Can you work these out from the drawing? Everything is in mm from the part's minimum corner. A direction names the side the tool comes from. Round coordinates to 2 decimals unless told otherwise and drop trailing zeros. Write each loop counter-clockwise with the first axis right and the second up, starting at its lowest first coordinate (ties: lowest second). Pieces come first, ordered by that corner, then holes. Notation, with made-up numbers: (-36.5, 34.25) -> (-5.5, 34.25) arc R12 cw to (-5.5, 49.25) -> close; hole circle Ø4 at (37, 25). An arc over 180 degrees is marked (long way). Answer as CSV lines item,"result".
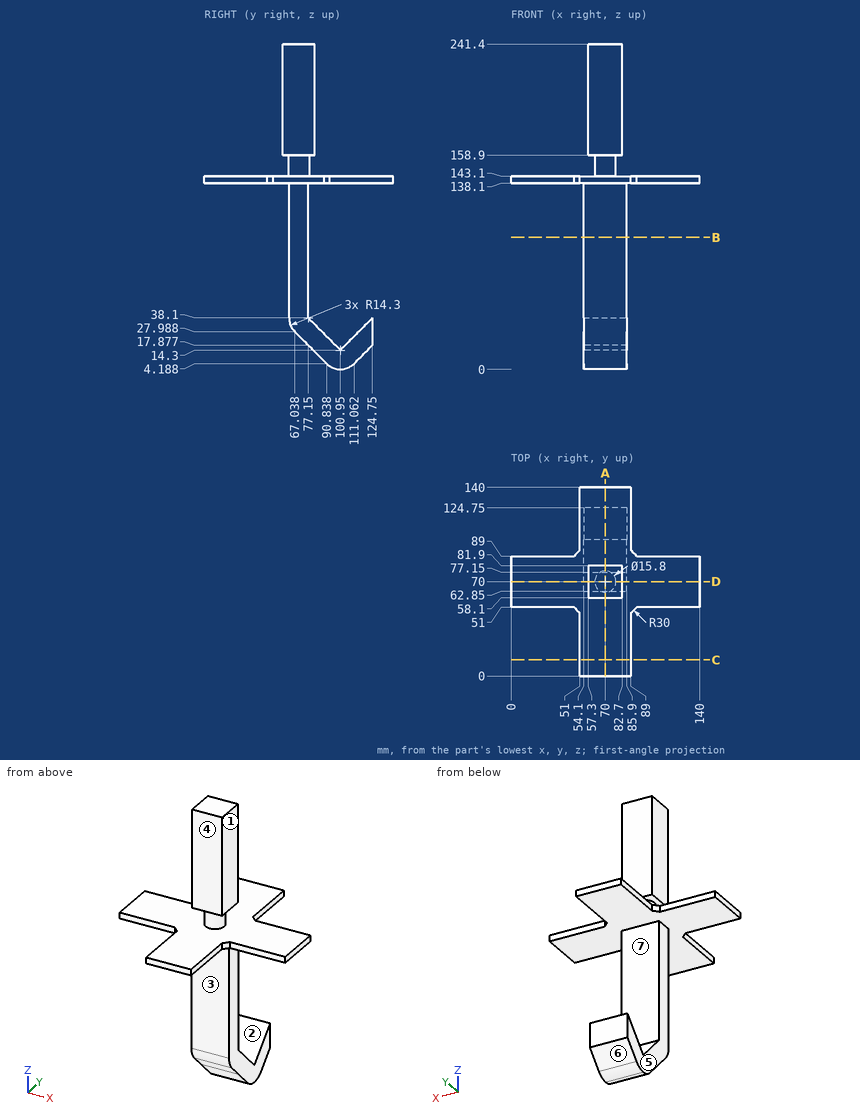
Item 1: If we mould it in two halves opening along Z, with no side actions, what happens to the marked faces 5, 6 and 7? For each: pulls with the +Z half, pulls with the -Z half, needs draft (parallel to the pull), parting line crosses it, or undercut.
Results found:
face 5,"needs draft"
face 6,"pulls with the -Z half"
face 7,"undercut"
Item 2: Will these pins go through, and if not, where does the flat tip stop? pin 1 (6 mm diameter, centred on y = 62, z = 43.5, fed in from +X); pin 2 (4 mm diameter, centred on x = 50.5, y = 20.5, fed in from -Z); pin 3 (4 mm diameter, centred on y = 127, z = 140.5, fed in from -X).
Results found:
pin 1,"stops at x = 85.9"
pin 2,"stops at z = 138.1"
pin 3,"stops at x = 51"
Item 3: Suppose I cut it at D-D, the plane y = 70. List the corners of the cut face in (x, z) for me, then the cut area to 3 significant figures.
Results found:
outline,"(0, 138.1) -> (54.1, 138.1) -> (54.1, 25.03) -> (85.9, 25.03) -> (85.9, 138.1) -> (140, 138.1) -> (140, 143.1) -> (77.9, 143.1) -> (77.9, 158.9) -> (82.7, 158.9) -> (82.7, 241.4) -> (57.3, 241.4) -> (57.3, 158.9) -> (62.1, 158.9) -> (62.1, 143.1) -> (0, 143.1) -> close"
area,"6,640 mm²"
Item 4: Suppose I cut it at A-A, the plane x = 70. List the corners of the cut face in (y, z) for me.
Results found:
outline,"(0, 138.1) -> (62.85, 138.1) -> (62.85, 38.1) arc R14.3 ccw to (67.04, 27.99) -> (77.15, 17.88) -> (90.84, 4.19) arc R14.3 ccw to (100.95, 0) arc R14.3 ccw to (111.06, 4.19) -> (124.75, 17.88) -> (124.75, 38.1) -> (100.95, 14.3) -> (77.15, 38.1) -> (77.15, 138.1) -> (140, 138.1) -> (140, 143.1) -> (77.9, 143.1) -> (77.9, 158.9) -> (81.9, 158.9) -> (81.9, 241.4) -> (58.1, 241.4) -> (58.1, 158.9) -> (62.1, 158.9) -> (62.1, 143.1) -> (0, 143.1) -> close"
Item 5: For the marked faces 1, 2, 3 and 4, which set-ups out of +Z, -Z, +X, -X, +Y, -Y let a thin tool reach every point of the face, with its end or its side?
Results found:
face 1,"+Z, +X, +Y, -Y"
face 2,"+X, -X"
face 3,"-Z, +X, -X, -Y"
face 4,"+Z, +X, -X, -Y"
Item 6: I need wall thicknesses on L1, parallel to X at y = 71.5, z = 39.5; L2, parallel to Z at x = 26.5, y = 67; L3, parallel to Y at x = 77.5, z = 204. Which ranges of each line are inside material? Lowest first, please.
Results found:
L1,"x = 54.1 to 85.9"
L2,"z = 138.1 to 143.1"
L3,"y = 58.1 to 81.9"
Item 7: Suppose I cut it at B-B, the plane z = 98. List the corners of the cut face in (x, y) for me, then the cut area to 3 significant figures.
Results found:
outline,"(54.1, 62.85) -> (85.9, 62.85) -> (85.9, 77.15) -> (54.1, 77.15) -> close"
area,"455 mm²"
Item 8: Suppose I cut it at C-C, the plane y = 12. List the corners of the cut face in (x, z) for me.
Results found:
outline,"(51, 138.1) -> (89, 138.1) -> (89, 143.1) -> (51, 143.1) -> close"
